Can you work these out from the model? Positions are in its coordinate system, mm. Face numbers are marked on the shaded views. A direction names the side the tool comes from. Give positions to 0.01 mm unless a question says otherwise; leave off trailing zeros. Use a Markdown table: item, result. Add a question column.
Autodesk Inventor part; units mm, degrees
ref_plane "FDT_MOUNT_XY" through (0, -22.75, 0) normal (0, 1, 0) x (-1, 0, 0)
ref_plane "FDT_MOUNT_YZ" through (0, -22.75, 0) normal (-1, 0, 0) x (0, 0, 1)
ref_plane "FDT_MOUNT_ZX" through (0, -22.75, 0) normal (0, 0, 1) x (0, 1, 0)
sketch "Sketch_19" plane through (0, 0, 0) normal (1, 0, 0) x (0, 1, 0)
  line L0 (-31.1, 0) -> (19.85, 0)
  line L1 (19.85, 0) -> (19.85, -4.672)
  line L2 (19.85, -4.672) -> (17.95, -6.1)
  line L3 (17.95, -6.1) -> (19.32, -6.1)
  line L4 (19.32, -6.1) -> (19.85, -6.3471)
  line L5 (19.85, -6.3471) -> (19.85, -6.5)
  line L6 (19.85, -6.5) -> (19.65, -6.7)
  line L7 (19.65, -6.7) -> (17.95, -6.7)
  line L8 (17.95, -6.7) -> (17.95, -11.75)
  line L9 (17.95, -11.75) -> (16.8819, -13.6)
  line L10 (16.8819, -13.6) -> (8.75, -13.6)
  line L11 (8.75, -13.6) -> (8.75, -13.9)
  line L12 (8.75, -13.9) -> (-19, -13.9)
  line L13 (-19, -13.9) -> (-19, -13.05)
  arc A0 (-19, -13.05) -> (-19.3, -13.35) centre (-19, -13.35) ccw
  line L14 (-19.3, -13.35) -> (-19.3, -13.9)
  line L15 (-19.3, -13.9) -> (-20.4, -13.9)
  line L16 (-20.4, -13.9) -> (-20.4, -13.225)
  line L17 (-20.4, -13.225) -> (-22.75, -13.225)
  line L18 (-22.75, -13.225) -> (-22.75, -10.4775)
  line L19 (-22.75, -10.4775) -> (-29.938, -10.4775)
  line L20 (-29.938, -10.4775) -> (-31.1, -9.3155)
  line L21 (-31.1, -9.3155) -> (-31.1, 0)
  line L22 (-31.1, 0) -> (19.85, 0)
revolve "Revolution1" add sketch "Sketch_19" angle 360 about axis through (0, -31.1, 0) along (0, -1, 0)
thread "Thread1"
sketch "Sketch_15" plane through (0, 19.85, 0) normal (0, 1, 0) x (1, 0, 0)
  line L0 (-24, -13.8564) -> (0, -27.7128)
  line L1 (0, -27.7128) -> (24, -13.8564)
  line L2 (24, -13.8564) -> (24, 13.8564)
  line L3 (24, 13.8564) -> (0, 27.7128)
  line L4 (0, 27.7128) -> (-24, 13.8564)
  line L5 (-24, 13.8564) -> (-24, -13.8564)
  line L6 (-12, -6.9282) -> (0, -13.8564)
  line L7 (0, -13.8564) -> (12, -6.9282)
  line L8 (12, -6.9282) -> (12, 6.9282)
  line L9 (12, 6.9282) -> (0, 13.8564)
  line L10 (0, 13.8564) -> (-12, 6.9282)
  line L11 (-12, 6.9282) -> (-12, -6.9282)
extrude "Extrusion1" cut sketch "Sketch_15" against normal blind 9.4
sketch "Sketch_16" plane through (0, 19.85, 0) normal (0, 1, 0) x (1, 0, 0)
  line L0 (-0.55, 5.9747) -> (-0.55, -5.9747)
  arc A0 (-0.55, -5.9747) -> (0.55, -5.9747) centre (0, 0) ccw
  line L1 (0.55, -5.9747) -> (0.55, 5.9747)
  arc A1 (0.55, 5.9747) -> (-0.55, 5.9747) centre (0, 0) ccw
extrude "Extrusion2" cut sketch "Sketch_16" against normal blind 1.2
sketch "Sketch_17" plane through (0, 0, 0) normal (1, 0, 0) x (0, 1, 0)
  line L0 (0, 0) -> (0, 41.4)
  line L1 (0, 41.4) -> (6.3, 41.4)
  line L2 (6.3, 41.4) -> (9.7347, 40.7944)
  arc A0 (9.9, 40.5974) -> (9.7347, 40.7944) centre (9.7, 40.5974) ccw
  line L3 (9.9, 40.5974) -> (9.9, 39.9)
  line L4 (9.9, 39.9) -> (7.9, 39.9)
  arc A1 (7.9, 39.9) -> (7.5, 39.5) centre (7.9, 39.5) ccw
  line L5 (7.5, 39.5) -> (7.5, 38.085)
  line L6 (7.5, 38.085) -> (8.6, 38.085)
  line L7 (8.6, 38.085) -> (8.7, 37.985)
  line L8 (8.7, 37.985) -> (8.7, 36.8)
  line L9 (8.7, 36.8) -> (9.9, 36.8)
  line L10 (9.9, 36.8) -> (9.9, 35.3)
  line L11 (9.9, 35.3) -> (10.25, 34.6938)
  line L12 (10.25, 34.6938) -> (10.25, 18.45)
  line L13 (10.25, 18.45) -> (7.5, 15.7)
  line L14 (7.5, 15.7) -> (7.5, 0)
  line L15 (7.5, 0) -> (0, 0)
  line L16 (0, 0) -> (0, 41.4)
revolve "Revolution2" add sketch "Sketch_17" angle 360 about axis through (0, 0, 0) along (0, 0, -1)
sketch "Sketch_18" plane through (0, 0, 0) normal (0, 0, 1) x (1, 0, 0)
  arc A0 (-7.5993, 2.5) -> (-7.5993, -2.5) centre (0, 0) ccw
  line L0 (-7.5993, -2.5) -> (7.5993, -2.5)
  arc A1 (7.5993, -2.5) -> (7.5993, 2.5) centre (0, 0) ccw
  line L1 (7.5993, 2.5) -> (-7.5993, 2.5)
extrude "Extrusion3" add sketch "Sketch_18" along normal blind 20.7
sketch "Sketch_5" plane through (0, 0, 0) normal (1, 0, 0) x (0, 1, 0)
  line L0 (0, 0) -> (0, 41.4)
  line L1 (0, 41.4) -> (6.3, 41.4)
  arc A0 (6.3, 41.4) -> (6, 41.1) centre (6.3, 41.1) ccw
  line L2 (6, 41.1) -> (6, 17.9)
  line L3 (6, 17.9) -> (3, 17.9)
  line L4 (3, 17.9) -> (3, 0)
  line L5 (3, 0) -> (0, 0)
  line L6 (0, 0) -> (0, 41.4)
revolve "Revolution3" cut sketch "Sketch_5" angle 360 about axis through (0, 0, 0) along (0, 0, -1)
sketch "Sketch7" plane through (0, -31.1, 0) normal (0, -1, 0) x (1, 0, 0)
  point P0 (0, 0)
hole "Hole1" at (0, -31.1, 0) direction (0, 1, 0) diameter 8 depth 37.1 countersink diameter 8.3464 countersink angle 60
ref_plane "FDT_MOUNT_XY" through (0, -22.75, 0) normal (0, 1, 0) x (-1, 0, 0)
ref_plane "FDT_MOUNT_YZ" through (0, -22.75, 0) normal (-1, 0, 0) x (0, 0, 1)
ref_plane "FDT_MOUNT_ZX" through (0, -22.75, 0) normal (0, 0, 1) x (0, 1, 0)
ref_plane "FDT_SCHLAUCH_XY" through (0, 0, 17.9) normal (0, 0, 1) x (1, 0, 0)
ref_plane "FDT_SCHLAUCH_YZ" through (0, 0, 17.9) normal (1, 0, 0) x (0, 1, 0)
ref_plane "FDT_SCHLAUCH_ZX" through (0, 0, 17.9) normal (0, 1, 0) x (0, 0, 1)
ref_plane "Zylinder_XY" through (0, -31.1, 0) normal (0, 1, 0) x (1, 0, 0)
ref_plane "Zylinder_YZ" through (0, -31.1, 0) normal (1, 0, 0) x (0, 0, -1)
ref_plane "Zylinder_ZX" through (0, -31.1, 0) normal (0, 0, -1) x (0, 1, 0)
ref_plane "anbau_XY" through (0, -22.75, 0) normal (0, 1, 0) x (1, 0, 0)
ref_plane "anbau_YZ" through (0, -22.75, 0) normal (1, 0, 0) x (0, 0, -1)
ref_plane "anbau_ZX" through (0, -22.75, 0) normal (0, 0, -1) x (0, 1, 0)
properties part number "193152 GRLA-1/2-QS-12-D"
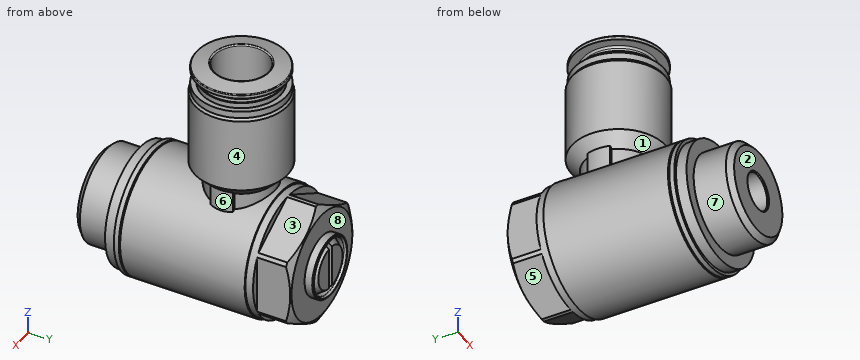
1. Will these pins go through, and if not, where does the flat tip stop? P1, Ø1.5, axis at x = -9.5, z = -2.5, coming from the +Y side; P2, Ø12, axis at x = -6.5, y = -5.5, coming from the -Z side; P3, Ø6, axis at y = 5.5, z = -6, coming from the +X side.
2. On a 3-axis mill with a long thin cutter (end or side, diameter ignored), from which of +Z, -Z, +X, -X, +Y, -Y can I reach the whole of each face in a straight line? I mean the marked faces 4, 5, 6, 7 and 8. Say none if no direction works.
3. If we mould it in two halves opening along Z, with no side actions, what happens to the marked faces 1, 2 and 3? For each: released by +Z, released by -Z, zero draft, split by the parting line, or undercut.
4. Please list where these lines run through material, in increasing order: line 1 along Y through (x, z) = (-12.25, -6); line 2 along Z through (x, y) = (2.25, -9); line 3 along X through (y, z) = (-4, 14). Write a range as [from, to].
Results below:
| question | item | result |
|---|---|---|
| 1 | P1 | y = 17.95 |
| 1 | P2 | z = -13.89 |
| 1 | P3 | x = 13.57 |
| 2 | face 4 | +Z |
| 2 | face 5 | -Z, -X, +Y |
| 2 | face 6 | +X |
| 2 | face 7 | -Y |
| 2 | face 8 | +Y |
| 3 | face 1 | undercut |
| 3 | face 2 | zero draft |
| 3 | face 3 | released by +Z |
| 4 | line 1 | [-20.4, -19.3], [-19, 8.75] |
| 4 | line 2 | [-13.72, -3.31], [3.31, 13.72], [17.48, 36.8], [39.9, 40.88] |
| 4 | line 3 | [-6.34, 6.34] |
